Source: CAD feature listing. Evaluate the final solid. Frame: model axes, mm. A direction names the side the tool comes from. Give positions to 0.01 mm unless a question says otherwise; leave off trailing zeros. Loops run counter-clockwise (first coordinate to the right, second up) from the corner with the lowest first, then second, coordinate; pieces in that order, holes last. Notation, with made-up numbers: (42, -3.75) -> (65, -3.75) arc R7 ccw to (65, 6.25) -> close; hole circle Ø8 at (-13, -7). An arc over 180 degrees is marked (long way). Return JSON: item names as keys, results as strings. Group by question number.
(1) Cut plane A-A on y = -30.5. Return loops of the section in (x, z), then the cut area to 3 significant figures.
(2) Access query for faces 1 (the face through (3, 10.16, -16)), 2 (the face through (3, -30, -42.926)), 3 (the face through (3, -48.311, -16)). Directions: +Z, -Z, +X, -X, +Y, -Y. A direction counts if a zero-diameter tool reaches every point of the face in a straight line with its end or side. Return the directions, or none.
(3) Cut plane C-C on x = 6. Return loops of the section in (y, z).
(4) Cut plane B-B on z = -25. Return loops of the section in (x, y), then the cut area to 3 significant figures.
(5) Pin query (flat end, axial travel): pin 1 (1.5 mm diameter, centred on x = 4.5, y = -41, fed in from -Z); pin 2 (8 mm diameter, centred on y = -17, z = -25, fed in from +X). Return the tip coordinate at first contact, or that it passes through.
(6) Ray query, line 1 (Y direction, x = 5.75, z = -27); line 2 (Z direction, x = 6, y = -42.5). Return the intervals inside material, ascending. Write a range as from..to.
```python
from build123d import *

# Parameters (mm, degrees)
F0_W     = 6.7056016997
F0_H     = 48.3108013868
F1_DEPTH = 10.16
F2_W     = 6.7056016997
F2_H     = 43.0277371144
F3_DEPTH = 10.16
F4_W     = 6.7056016997
F4_H     = 42.9259994364
F5_DEPTH = 10.16
F6_W     = 6.7056016997
F6_H     = 58.4708013868
F7_DEPTH = 10.16
F8_W     = 6.7056016997
F8_H     = 10.16
F9_DEPTH = 10.16


with BuildPart() as f1:
    # F0 (on Top) → F1 (new body)
    with BuildSketch(Plane.XY):
        with Locations((3.3528008498, -24.1554006934)):
            Rectangle(F0_W, F0_H)
    extrude(amount=F1_DEPTH)

    # F2 (on face) → F3 (join)
    with BuildSketch(Plane(origin=(0, 0, 0), x_dir=(-1, 0, 0), z_dir=(0, 1, 0))):
        with Locations((-3.3528008498, -11.3538685572)):
            Rectangle(F2_W, F2_H)
    extrude(amount=F3_DEPTH)

    # F4 (on face) → F5 (join)
    with BuildSketch(Plane.XZ.offset(48.3108013868)):
        with Locations((3.3528008498, -11.3029997182)):
            Rectangle(F4_W, F4_H)
    extrude(amount=F5_DEPTH)

    # F6 (on face) → F7 (join)
    with BuildSketch(Plane(origin=(0, 0, -32.7659994364), x_dir=(1, 0, 0), z_dir=(0, 0, -1))):
        with Locations((3.3528008498, 29.2354006934)):
            Rectangle(F6_W, F6_H)
    extrude(amount=F7_DEPTH)

    # F8 (on face) → F9 (join)
    with BuildSketch(Plane(origin=(0, 0, -32.8677371144), x_dir=(1, 0, 0), z_dir=(0, 0, -1))):
        with Locations((3.3528008498, -5.08)):
            Rectangle(F8_W, F8_H)
    extrude(amount=F9_DEPTH)


solid = f1.part
```
Answers:
{
 "1": {"outline": "(0, -42.93) -> (6.71, -42.93) -> (6.71, -32.77) -> (0, -32.77) -> close; (0, 0) -> (6.71, 0) -> (6.71, 10.16) -> (0, 10.16) -> close", "area": "136 mm²"},
 "2": {"face 1": "+Z, -Z, +X, -X, +Y", "face 2": "-Z, +X, -X, -Y", "face 3": "+X, -X"},
 "3": {"outline": "(-58.47, -42.93) -> (0, -42.93) -> (0, -43.03) -> (10.16, -43.03) -> (10.16, 10.16) -> (-58.47, 10.16) -> close; hole (-48.31, -32.77) -> (0, -32.77) -> (0, 0) -> (-48.31, 0) -> close"},
 "4": {"outline": "(0, -58.47) -> (6.71, -58.47) -> (6.71, -48.31) -> (0, -48.31) -> close; (0, 0) -> (6.71, 0) -> (6.71, 10.16) -> (0, 10.16) -> close", "area": "136 mm²"},
 "5": {"pin 1": "z = -42.93", "pin 2": "through"},
 "6": {"line 1": "-58.47..-48.31, 0..10.16", "line 2": "-42.93..-32.77, 0..10.16"}
}
